Can you work these out from the model? Positions are in its coordinate system, mm. Face numbers are marked on the shaded views. A direction names the side the tool comes from. Coordinates: 2 decimals unless noted, no trailing zeros. Order: outer loops, then holes, each group sorted by start corner. A loop starts at its lowest first (then second) coordinate and runs counter-clockwise, first axis right, second up.
```python
from build123d import *

# Parameters (mm, degrees)
F0_W     = 179
F0_H     = 12
F0_W_2   = 138
F0_H_2   = 40
F0_W_3   = 40
F0_H_3   = 120
F0_W_4   = 92
F0_W_5   = 12
F0_H_4   = 90
F0_H_5   = 180
F0_W_6   = 87
F0_H_6   = 92
F0_W_7   = 26
F0_H_7   = 142
F0_H_8   = 136
F0_W_8   = 228
F0_H_9   = 18
F0_H_10  = 20
F0_W_9   = 20
F1_DEPTH = 5
F2_DEPTH = 277
F3_W     = 40
F3_H     = 120
F3_H_2   = 180
F4_DEPTH = 27
F6_DEPTH = 1195.001


with BuildPart() as f1:
    # F0 (on Top) → F1 (new body)
    with BuildSketch(Plane.XY):
        with Locations((1040.5, 269)):
            Rectangle(F0_W, F0_H)
        Polygon((794, 408), (794, 420), (669, 420), (669, 515), (652, 515), (652, 503), (657, 503), (657, 408), align=None)
        with Locations((392, -5)):
            Rectangle(F0_W_2, F0_H_2)
        Polygon((1130, 350), (1130, 530), (1130, 780), (806, 780), (806, 691), (832, 691), (832, 549), (806, 549), (806, 385), (806, 293), (806, 275), (839, 275), (859, 275), (951, 275), (1130, 275), align=None)
        with Locations((-5, 547.5)):
            Rectangle(F0_W_3, F0_H_3)
        with Locations((-5, 247.5)):
            Rectangle(F0_W_3, F0_H_3)
        Polygon((15, 487.5), (-25, 487.5), (-25, 307.5), (15, 307.5), (15, 382.1609020233), (15, 391.5), (15, 403.5), align=None)
        Polygon((15, 187.5), (-25, 187.5), (-25, -25), (323, -25), (323, 15), (15, 15), align=None)
        Polygon((1130, 15), (1130, 263), (951, 263), (859, 263), (839, 263), (839, 243), (839, 151), (839, 15), align=None)
        with Locations((905, 269)):
            Rectangle(F0_W_4, F0_H)
        Polygon((364.8940163038, 391.5), (243, 391.5), (243, 382.5), (364.8667633533, 382.5), align=None)
        Polygon((473, 780), (461, 780), (461, 498.5), (473, 498.5), (473, 503), (473, 515), align=None)
        with Locations((467, 453.5)):
            Rectangle(F0_W_5, F0_H_4)
        Polygon((243, 426.5), (243, 403.5), (364.9303535711, 403.5), (365, 426.5), align=None)
        Polygon((473, 503), (473, 498.5), (473, 408.5), (473, 386.5), (473, 296.5), (473, 275), (653, 275), (670, 275), (794, 275), (794, 293), (794, 385), (794, 408), (657, 408), (657, 503), (652, 503), (560, 503), align=None)
        with Locations((1150, 440)):
            Rectangle(F0_W_3, F0_H_5)
        Polygon((665, 263), (665, 15), (827, 15), (827, 151), (827, 243), (827, 263), (806, 263), (794, 263), align=None)
        with Locations((516.5, 509)):
            Rectangle(F0_W_6, F0_H)
        with Locations((467, 341.5)):
            Rectangle(F0_W_5, F0_H_4)
        Polygon((15, 382.1609020233), (15, 307.5), (15, 187.5), (15, 15), (323, 15), (461, 15), (461, 198.5), (435, 198.5), (435, 262.5), (461, 262.5), (461, 296.5), (461, 386.5), (461, 391.5), (365, 391.5), (364.8940163038, 391.5), (364.8667633533, 382.5), (243, 382.5), (243, 391.5), (15, 391.5), align=None)
        Polygon((1170, 530), (1170, 820), (-25, 820), (-25, 607.5), (15, 607.5), (15, 780), (461, 780), (473, 780), (794, 780), (806, 780), (1130, 780), (1130, 530), align=None)
        with Locations((833, 197)):
            Rectangle(F0_W_5, F0_H_6)
        Polygon((461, 198.5), (461, 15), (473, 15), (473, 275), (473, 296.5), (461, 296.5), (461, 262.5), (435, 262.5), (435, 198.5), align=None)
        Polygon((794, 420), (794, 780), (473, 780), (473, 515), (560, 515), (652, 515), (669, 515), (669, 420), align=None)
        with Locations((819, 620)):
            Rectangle(F0_W_7, F0_H_7)
        with Locations((606, 509)):
            Rectangle(F0_W_4, F0_H)
        with Locations((833, 83)):
            Rectangle(F0_W_5, F0_H_8)
        Polygon((653, 275), (653, 15), (665, 15), (665, 263), (794, 263), (794, 275), (670, 275), align=None)
        Polygon((1170, -25), (1170, 350), (1130, 350), (1130, 275), (1130, 263), (1130, 15), (839, 15), (827, 15), (665, 15), (653, 15), (473, 15), (461, 15), (461, -25), align=None)
        with Locations((800, 339)):
            Rectangle(F0_W_5, F0_H_6)
        with Locations((129, 397.5)):
            Rectangle(F0_W_8, F0_H)
        with Locations((800, 284)):
            Rectangle(F0_W_5, F0_H_9)
        Polygon((806, 691), (806, 780), (794, 780), (794, 420), (794, 408), (794, 385), (806, 385), (806, 549), align=None)
        with Locations((833, 253)):
            Rectangle(F0_W_5, F0_H_10)
        Polygon((839, 263), (839, 275), (806, 275), (806, 263), (827, 263), align=None)
        with Locations((849, 269)):
            Rectangle(F0_W_9, F0_H)
        Polygon((365, 403.5), (364.9303535711, 403.5), (364.8940163038, 391.5), (365, 391.5), (461, 391.5), (461, 386.5), (473, 386.5), (473, 408.5), (461, 408.5), (461, 403.5), align=None)
        Polygon((364.9303535711, 403.5), (243, 403.5), (243, 391.5), (364.8940163038, 391.5), align=None)
        with Locations((800, 269)):
            Rectangle(F0_W_5, F0_H)
        Polygon((15, 780), (15, 607.5), (15, 487.5), (15, 403.5), (243, 403.5), (243, 426.5), (365, 426.5), (364.9303535711, 403.5), (365, 403.5), (461, 403.5), (461, 408.5), (461, 498.5), (461, 780), align=None)
    extrude(amount=F1_DEPTH)

    # F0 (on Top) → F2 (join)
    with BuildSketch(Plane.XY):
        Polygon((15, 187.5), (-25, 187.5), (-25, -25), (323, -25), (323, 15), (15, 15), align=None)
        with Locations((392, -5)):
            Rectangle(F0_W_2, F0_H_2)
        Polygon((1170, -25), (1170, 350), (1130, 350), (1130, 275), (1130, 263), (1130, 15), (839, 15), (827, 15), (665, 15), (653, 15), (473, 15), (461, 15), (461, -25), align=None)
        with Locations((833, 83)):
            Rectangle(F0_W_5, F0_H_8)
        Polygon((653, 275), (653, 15), (665, 15), (665, 263), (794, 263), (794, 275), (670, 275), align=None)
        Polygon((461, 198.5), (461, 15), (473, 15), (473, 275), (473, 296.5), (461, 296.5), (461, 262.5), (435, 262.5), (435, 198.5), align=None)
        Polygon((15, 487.5), (-25, 487.5), (-25, 307.5), (15, 307.5), (15, 382.1609020233), (15, 391.5), (15, 403.5), align=None)
        with Locations((129, 397.5)):
            Rectangle(F0_W_8, F0_H)
        Polygon((243, 426.5), (243, 403.5), (364.9303535711, 403.5), (365, 426.5), align=None)
        Polygon((364.9303535711, 403.5), (243, 403.5), (243, 391.5), (364.8940163038, 391.5), align=None)
        Polygon((364.8940163038, 391.5), (243, 391.5), (243, 382.5), (364.8667633533, 382.5), align=None)
        Polygon((365, 403.5), (364.9303535711, 403.5), (364.8940163038, 391.5), (365, 391.5), (461, 391.5), (461, 386.5), (473, 386.5), (473, 408.5), (461, 408.5), (461, 403.5), align=None)
        Polygon((473, 780), (461, 780), (461, 498.5), (473, 498.5), (473, 503), (473, 515), align=None)
        with Locations((516.5, 509)):
            Rectangle(F0_W_6, F0_H)
        Polygon((794, 408), (794, 420), (669, 420), (669, 515), (652, 515), (652, 503), (657, 503), (657, 408), align=None)
        Polygon((806, 691), (806, 780), (794, 780), (794, 420), (794, 408), (794, 385), (806, 385), (806, 549), align=None)
        with Locations((833, 253)):
            Rectangle(F0_W_5, F0_H_10)
        with Locations((849, 269)):
            Rectangle(F0_W_9, F0_H)
        Polygon((839, 263), (839, 275), (806, 275), (806, 263), (827, 263), align=None)
        with Locations((800, 269)):
            Rectangle(F0_W_5, F0_H)
        with Locations((800, 284)):
            Rectangle(F0_W_5, F0_H_9)
        with Locations((1040.5, 269)):
            Rectangle(F0_W, F0_H)
        Polygon((1170, 530), (1170, 820), (-25, 820), (-25, 607.5), (15, 607.5), (15, 780), (461, 780), (473, 780), (794, 780), (806, 780), (1130, 780), (1130, 530), align=None)
        with Locations((819, 620)):
            Rectangle(F0_W_7, F0_H_7)
    extrude(amount=F2_DEPTH)

    # F3 (on face) → F4 (join)
    with BuildSketch(Plane.XY.offset(277)):
        with Locations((-5, 547.5)):
            Rectangle(F3_W, F3_H)
        with Locations((-5, 397.5)):
            Rectangle(F3_W, F3_H_2)
        with Locations((-5, 247.5)):
            Rectangle(F3_W, F3_H)
        with Locations((1150, 440)):
            Rectangle(F3_W, F3_H_2)
    extrude(amount=-F4_DEPTH)

    # F5 (on face) → F6 (cut, through all)
    with BuildSketch(Plane(origin=(-25, 0, 0), x_dir=(0, -1, 0), z_dir=(-1, 0, 0))):
        Polygon((-669.6397058824, 277), (-397.5, 496), (-820, 496), (-820, 277), align=None)
        Polygon((-820, 156), (-669.6397058824, 277), (-820, 277), align=None)
        Polygon((25, 496), (-397.5, 496), (-125.3602941176, 277), (25, 277), align=None)
        Polygon((25, 277), (-125.3602941176, 277), (25, 156), align=None)
    extrude(amount=-F6_DEPTH, mode=Mode.SUBTRACT)


solid = f1.part
```
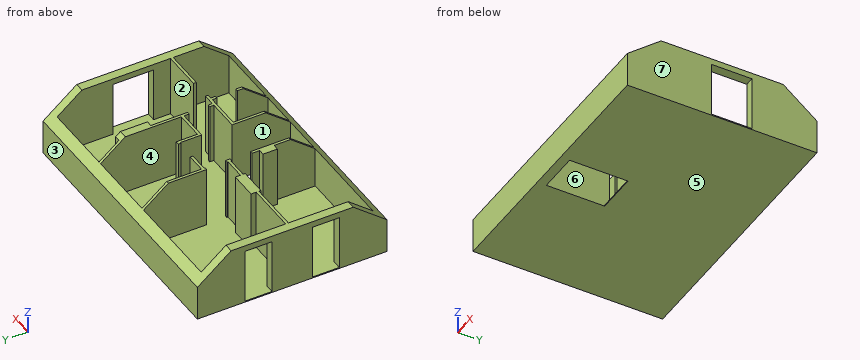
1. On a 3-axis mill with a long thin cutter (end or side, diameter ignored), from which of +Z, -Z, +X, -X, +Y, -Y can I reach the whole of each face in a straight line? I mean the marked faces 1, 2 and 3. Say none if no direction works.
Completed:
face 1: +Z, -Z
face 2: +Z
face 3: +Z, -Z, +X, -X, +Y
2. Imagine slicing it at A-A on y = 461.5. Please give me the cut outline in (x, z).
Completed:
outline: (-25, 0) - (1170, 0) - (1170, 5) - (806, 5) - (806, 277) - (794, 277) - (794, 5) - (669, 5) - (669, 277) - (657, 277) - (657, 5) - (15, 5) - (15, 277) - (-25, 277) - close; (1130, 250) - (1170, 250) - (1170, 277) - (1130, 277) - close
3. I'm going to push flat-ended pins straight in: pin 1 (3 mm diameter, centred on y = 438, z = 161.5, fed in from +X); pin 2 (6 mm diameter, centred on x = 686, z = 199, fed in from +Y); pin 3 (2 mm diameter, centred on x = 249.5, y = 465.5, fed in from +Z). Where does each tip first touch, or does it pass through?
Completed:
pin 1: stops at x = 806
pin 2: stops at y = 420
pin 3: stops at z = 5
4. Please list where these lines run through material, in increasing order: probe 1 along Y at (x, z) = (1083.5, 62); probe 2 along Y at (x, z) = (733.5, 152.5); probe 3 along X at (y, z) = (266, 64.5).
Completed:
probe 1: y = -25 to 15, 263 to 275, 780 to 820
probe 2: y = -25 to 15, 263 to 275, 408 to 420, 780 to 820
probe 3: x = 461 to 473, 653 to 859, 951 to 1170
5. Thinking about a two-plate mould opening in X: for the marked faces 4, 5, 6 and 7, which applies, pulls with the +X half, pulls with the -X half, needs draft (parallel to the pull), parting line crosses it, or undercut?
Completed:
face 4: undercut
face 5: needs draft
face 6: undercut
face 7: pulls with the +X half
6. Imagine slicing it at B-B on x = 513.5. Please give me the cut outline in (y, z), then the cut area to 3 significant figures.
Completed:
outline: (-25, 0) - (15, 0) - (15, 188.19) - (-25, 156) - close; (275, 0) - (820, 0) - (820, 156) - (780, 188.19) - (780, 5) - (515, 5) - (515, 277) - (503, 277) - (503, 5) - (275, 5) - close
area: 19,600 mm2
7. Imagine slicing it at D-D on y = 754. Please give me the cut outline in (x, z).
Completed:
outline: (-25, 0) - (1170, 0) - (1170, 209.11) - (1130, 209.11) - (1130, 5) - (806, 5) - (806, 209.11) - (794, 209.11) - (794, 5) - (473, 5) - (473, 209.11) - (461, 209.11) - (461, 5) - (15, 5) - (15, 209.11) - (-25, 209.11) - close
8. Imagine slicing it at C-C on x = 101.5. Please give me the cut outline in (y, z), then the cut area to 3 significant figures.
Completed:
outline: (-25, 0) - (820, 0) - (820, 156) - (780, 188.19) - (780, 5) - (403.5, 5) - (403.5, 277) - (391.5, 277) - (391.5, 5) - (15, 5) - (15, 188.19) - (-25, 156) - close
area: 20,900 mm2
